Build history of the part. All positions in model axes, mm. A direction names the side the tool comes from. Round coordinates to 2 decimals unless told otherwise and drop trailing zeros. Write each loop counter-clockwise with the first axis right and the second up, starting at its lowest first coordinate (ties: lowest second). Pieces come first, ordered by that corner, then holes. Notation, with made-up numbers: (-33, 1) - (15, 1) arc R19 ccw to (15, 24) - close; hole circle Ø6 at (53.25, 3). An arc over 180 degrees is marked (long way). Write each question's results on one line, items separated by ' | '.
from build123d import *

# Parameters (mm, degrees)
ESBO_O8_R             = 20
CORTE_EXTRUS_O1_DEPTH = 140
ESBO_O9_R             = 5
CORTE_EXTRUS_O2_DEPTH = 20


with BuildPart() as part:
    # Esboço1 → Revolução1 (revolve)
    with BuildSketch(Plane.XY):
        with BuildLine():
            Line((-67.020117474, 0), (-94.010110831, 0))
            Line((-94.010110831, 0), (-94.010110831, 70))
            Line((-94.010110831, 70), (-84.391943284, 70))
            ThreePointArc((-84.391943284, 70), (-77.378586892, 48.382660787), (-59.010110831, 35))
            Line((-59.010110831, 35), (60.989889169, 35))
            Line((60.989889169, 35), (60.989889169, 0))
            Line((60.989889169, 0), (-67.020117474, 0))
        make_face()
    revolve(axis=Axis((-67.020117474, 0, 0), (-1, 0, 0)))

    # Esboço8 → Corte-extrusão1 (cut)
    with BuildSketch(Plane(origin=(60.989889169, 0, 0), x_dir=(0, 0, -1), z_dir=(1, 0, 0))):
        Circle(ESBO_O8_R)
    extrude(amount=-CORTE_EXTRUS_O1_DEPTH, mode=Mode.SUBTRACT)

    # Esboço9 → Corte-extrusão2 (cut)
    with BuildSketch(Plane(origin=(60.989889169, 0, 0), x_dir=(0, 0, -1), z_dir=(1, 0, 0))):
        with Locations((0, 27.5)):
            Circle(ESBO_O9_R)
        with Locations((27.5, 0)):
            Circle(ESBO_O9_R)
        with Locations((-27.5, 0)):
            Circle(ESBO_O9_R)
        with Locations((0, -27.5)):
            Circle(ESBO_O9_R)
    extrude(amount=-CORTE_EXTRUS_O2_DEPTH, mode=Mode.SUBTRACT)


solid = part.part
(1) Two-plate mould, pull along Y, no slides. Class faces 3 (the flat face through (60.99, 15, 15)), 4 (the flat face through (40.99, 0, 28)), 5 (the cylindrical face through (-89.134, -55.55, 42.594)), 6 (the cylindrical face through (51.13, 0.22, 32.495)): released by +Y, released by -Y, zero draft, split by the parting line, or undercut.
Worked answers:
face 3: zero draft | face 4: undercut | face 5: split by the parting line | face 6: undercut
(2) Tool access for faces 1 (the cylindrical face through (51.13, 22.62, 1.08)), 2 (the flat face through (-94.01, 1, -1)): list every direction of +Z, -Z, +X, -X, +Y, -Y with a clear straight run to the whole face (end or side of a thin tool).
Worked answers:
face 1: +X | face 2: +Z, -Z, -X, +Y, -Y
(3) Slice it at D-D, the plane x = -68. Write the cut outline in (y, z).
Worked answers:
outline: circle Ø78.73 at (0, 0); hole circle Ø40 at (0, 0)
(4) Slice it at B-B, the plane x = 32.5. Write the cut outline in (y, z).
Worked answers:
outline: circle Ø70 at (0, 0); hole circle Ø40 at (0, 0)
(5) Drill centre lines: probe 1 along Y at (x, z) = (54.75, 0); probe 2 along Y at (x, z) = (-4.5, 0); probe 3 along Y at (x, z) = (47.5, 27.5). Where is each one in solid material? Low to high. Write a range as [from, to].
Worked answers:
probe 1: y = [-35, -32.5], [-22.5, -20], [20, 22.5], [32.5, 35] | probe 2: y = [-35, -20], [20, 35] | probe 3: y = [-21.65, -5], [5, 21.65]
(6) Slice it at A-A, the plane z = 0. Write the cut outline in (x, y), and give its area (3 significant figures).
Worked answers:
outline: (-94.01, -70) - (-84.39, -70) arc R36.82 cw to (-59.01, -35) - (60.99, -35) - (60.99, -32.5) - (40.99, -32.5) - (40.99, -22.5) - (60.99, -22.5) - (60.99, -20) - (-79.01, -20) - (-79.01, 20) - (60.99, 20) - (60.99, 22.5) - (40.99, 22.5) - (40.99, 32.5) - (60.99, 32.5) - (60.99, 35) - (-59.01, 35) arc R36.82 cw to (-84.39, 70) - (-94.01, 70) - close | area: 6,000 mm2
(7) Flat gauge pins, fed straight in: pin 1 Ø4 at (x, y) = (-55, -15.5) entering from -Z; pin 2 Ø3 at (y, z) = (25.5, -1) entering from +X; pin 3 Ø1.5 at (x, y) = (-68, -34) entering from -Z. Where does each tip first touch, or does it go through?
Worked answers:
pin 1: stops at z = -32.29 | pin 2: stops at x = 40.99 | pin 3: stops at z = -21.41
